```python
from build123d import *

# Parameters (mm, degrees)
BOSS_EXTRUDE1_DEPTH = 50.8
BOSS_EXTRUDE3_DEPTH = 25.4


# Read off the part's stored shape, not the designer's step: Boss-Extrude3
with BuildPart() as part:
    # Sketch1 → Boss-Extrude1 (new body)
    with BuildSketch(Plane.XY):
        with BuildLine():
            Line((3.175, 0), (0, 0))
            Line((0, 0), (0, -387.1625))
            ThreePointArc((0, -387.1625), (1.464466094, -390.698033906), (5, -392.1625))
            Line((5, -392.1625), (50.8, -392.1625))
            Line((50.8, -392.1625), (50.8, -388.9875))
            Line((50.8, -388.9875), (8.175, -388.9875))
            ThreePointArc((8.175, -388.9875), (4.639466094, -387.523033906), (3.175, -383.9875))
            Line((3.175, -383.9875), (3.175, 0))
        make_face()
    extrude(amount=BOSS_EXTRUDE1_DEPTH)

    # Boss-Extrude3 outline → Boss-Extrude3 (add)
    with BuildSketch(Plane(origin=(0, -194.49375, 0), x_dir=(1, 0, 0), z_dir=(0, 1, 0))):
        with BuildLine():
            Line((11.147027194, 0), (7.338766309, 0))
            Line((7.338766309, 0), (3.175, 0))
            Line((3.175, 0), (3.175, -25.4))
            ThreePointArc((3.175, -25.4), (5.214810239, -12.089165902), (11.147027194, 0))
        make_face()
        with BuildLine():
            ThreePointArc((7.338766309, -50.8), (95.25, -25.4), (7.338766309, 0))
            Line((7.338766309, 0), (11.147027194, 0))
            ThreePointArc((11.147027194, 0), (60.935834098, 17.010189761), (92.075, -25.4))
            ThreePointArc((92.075, -25.4), (60.935834098, -67.810189761), (11.147027194, -50.8))
            Line((11.147027194, -50.8), (7.338766309, -50.8))
        make_face()
        with BuildLine():
            Line((3.175, -50.8), (7.338766309, -50.8))
            Line((7.338766309, -50.8), (11.147027194, -50.8))
            ThreePointArc((11.147027194, -50.8), (5.214810239, -38.710834098), (3.175, -25.4))
            Line((3.175, -25.4), (3.175, -50.8))
        make_face()
    extrude(amount=BOSS_EXTRUDE3_DEPTH)


solid = part.part
```
Read the model definition and answer for the solid it produces. Units are mm, in the model's axes. A direction names the side the tool comes from. Round coordinates to 2 decimals unless told otherwise and drop trailing zeros. Write each loop counter-clockwise with the first axis right and the second up, starting at its lowest first coordinate (ties: lowest second). Pieces come first, ordered by that corner, then holes. Notation, with made-up numbers: (45.5, 12.5) -> (59.5, 12.5) arc R20 cw to (59.5, 22.5) -> close; hole circle Ø7 at (1, 74). An arc over 180 degrees is marked (long way). Answer in a Markdown table with one row per item. Add a question column.
1) Find section C-C, the plane y = -180. Determine the outline of the cut face in (x, z) (3 decimals), and give its area (3 significant figures).
2) Find section A-A, the plane x = 79. Determine the outline of the cut face in (y, z).
3) Which of the six approach directions +Z, -Z, +X, -X, +Y, -Y give full straight-line access (tool end or side, diameter ignored) to faces 1 (the face through (95.22, -181.97, 27.12)), 2 (the face through (80, -194.494, 57))?
4) Consider line 1 (X direction, y = -16, z = 15) (3 decimals); line 2 (Y direction, x = 39.5, z = 35); line 3 (Z direction, x = 42, y = -175). Determine where each line is inside the solid, lowest interval first.
5) Determine the mould class of faces 3 (the face through (80, -169.094, 57)), 4 (the face through (3.175, -291, 25)), 5 (the face through (3.175, -86, 25)) for opening direction Y: pulls with the +Y half, pulls with the -Y half, needs draft (parallel to the pull), parting line crosses it, or undercut.
6) Given P1, Ø13, axis at x = 36.5, z = 36, coming from the +Y side; P2, Ø1.5, axis at y = -189.5, z = 22.5, coming from the +X side; P3, Ø1, axis at y = -167.5, z = 48.5, coming from the +X side (3 decimals), each flat-ended and moving along its own axis, determine where each tip first touches the part or whether it passes through.
7) Find section D-D, the plane x = 37. Determine the outline of the cut face in (y, z).
8) Find section B-B, the plane z = 16.5. Determine the outline of the cut face in (x, y) (1 decimal).
Findings below:
| question | item | result |
|---|---|---|
| 1 | outline | (0, 0) -> (7.339, 0) arc R47.625 ccw (long way) to (7.339, 50.8) -> (0, 50.8) -> close; hole circle Ø88.9 at (47.625, 25.4) |
| 1 | area | 1,040 mm² |
| 2 | outline | (-194.49, -10.43) -> (-169.09, -10.43) -> (-169.09, -6.09) -> (-194.49, -6.09) -> close; (-194.49, 56.89) -> (-169.09, 56.89) -> (-169.09, 61.23) -> (-194.49, 61.23) -> close |
| 3 | face 1 | +Y, -Y |
| 3 | face 2 | +Z, -Z, +X |
| 4 | line 1 | 0 to 3.175 |
| 4 | line 2 | -392.16 to -388.99 |
| 4 | line 3 | -21.89 to -18.69, 69.49 to 72.69 |
| 5 | face 3 | pulls with the +Y half |
| 5 | face 4 | undercut |
| 5 | face 5 | needs draft |
| 6 | P1 | y = -388.99 |
| 6 | P2 | x = 95.2 |
| 6 | P3 | x = 3.175 |
| 7 | outline | (-392.16, 0) -> (-388.99, 0) -> (-388.99, 50.8) -> (-392.16, 50.8) -> close; (-194.49, -21.02) -> (-169.09, -21.02) -> (-169.09, -17.76) -> (-194.49, -17.76) -> close; (-194.49, 68.56) -> (-169.09, 68.56) -> (-169.09, 71.82) -> (-194.49, 71.82) -> close |
| 8 | outline | (0, -387.2) arc R5 ccw to (5, -392.2) -> (50.8, -392.2) -> (50.8, -389) -> (8.2, -389) arc R5 cw to (3.2, -384) -> (3.2, -194.5) -> (4.1, -194.5) -> (4.1, -169.1) -> (3.2, -169.1) -> (3.2, 0) -> (0, 0) -> close; (91.2, -194.5) -> (94.4, -194.5) -> (94.4, -169.1) -> (91.2, -169.1) -> close |
